Read the model definition and answer for the solid it produces. Units are mm, in the model's axes. Give positions to 0.01 mm unless a question says otherwise; leave off trailing zeros. Write each loop counter-clockwise with the first axis right and the second up, starting at its lowest first coordinate (ties: lowest second). Pieces come first, ordered by that corner, then holes. Notation, with made-up numbers: (4.25, 46.5) -> (47.25, 46.5) arc R10 cw to (47.25, 62.5) -> close; hole circle Ø6 at (-23, 53.25). An arc over 180 degrees is marked (long way). Put each result on its own line as item: value. Start each with the question number.
from build123d import *

# Parameters (mm, degrees)
SKETCH1_R           = 3.3020000000000405
BOSS_EXTRUDE1_DEPTH = 1.5875
SKETCH2_R           = 12.7
CUT_EXTRUDE1_DEPTH  = 164.69798740092241
CUT_EXTRUDE2_DEPTH  = 399.2312021708926
CUT_EXTRUDE3_DEPTH  = 399.2322845032196


with BuildPart() as part:
    # Sketch1 → Boss-Extrude1 (new body)
    with BuildSketch(Plane(origin=(-4.904e-14, 229.6997332170858, -328.0452161431734), x_dir=(1, 7e-17, -1e-16), z_dir=(0, -0.5735764363510497, 0.8191520442889892))):
        with BuildLine():
            Line((356.2998896252525, 70.55163741306428), (376.9254322382814, 80.82199071424783))
            ThreePointArc((376.9254322382814, 80.82199071424783), (382.63309358192566, 97.85145347695013), (365.6036308192234, 103.55911482059432))
            Line((365.6036308192234, 103.55911482059432), (344.97808820619434, 93.28876151941097))
            Line((344.97808820619434, 93.28876151941097), (356.2998896252525, 70.55163741306428))
        make_face()
        with Locations(Location((375.5277422986924, 94.3133905334945, 0), (0, 0, 270))):
            Circle(SKETCH1_R, mode=Mode.SUBTRACT)
    extrude(amount=BOSS_EXTRUDE1_DEPTH)

    # Sketch2 → Cut-Extrude1 (cut, through all)
    with BuildSketch(Plane(origin=(364.35174229869244, 343.62540364794484, -135.39966553044988), x_dir=(-0.9960075449626111, 0.027318171664055604, 0.08498639817338811), z_dir=(-0.0892690897094424, -0.3047987291070713, -0.9482240053685426))):
        Circle(SKETCH2_R)
    extrude(amount=CUT_EXTRUDE1_DEPTH, mode=Mode.SUBTRACT)

    # Sketch3 → Cut-Extrude2 (cut, through all)
    with BuildSketch(Plane(origin=(-4.885e-14, 228.78918062437845, -326.7448122728647), x_dir=(1, 7e-17, -1e-16), z_dir=(0, -0.5735764363510497, 0.8191520442889892))):
        with BuildLine():
            Line((359.8287026568516, 100.68352732070262), (358.4382239247449, 99.99114758047237))
            Line((358.4382239247449, 99.99114758047237), (360.8702636019665, 72.82742507790554))
            add(Edge.make_bspline(
                [(360.8702636019665, 72.82742507790554), (368.2083080665997, 89.03003410456597), (359.8287026568516, 100.68352732070262)],
                knots=[4.218717035603661, 4.218717035603661, 4.218717035603661, 5.696136664554478, 5.696136664554478, 5.696136664554478], degree=2, weights=[1, 0.7393379003717987, 1]))
        make_face()
    extrude(amount=-CUT_EXTRUDE2_DEPTH, mode=Mode.SUBTRACT)

    # Sketch4 → Cut-Extrude3 (cut, through all)
    with BuildSketch(Plane(origin=(-4.904e-14, 229.6997332170858, -328.0452161431734), x_dir=(-1, -7e-17, 1e-16), z_dir=(0, 0.5735764363510497, -0.8191520442889892))):
        with BuildLine():
            Line((-361.6174533376439, 73.19948329292563), (-360.8702636019665, 72.82742507790549))
            Line((-360.8702636019665, 72.82742507790549), (-363.361378453228, 81.54873685940132))
            add(Edge.make_bspline(
                [(-363.361378453228, 81.54873685940132), (-363.00233152155374, 77.177344146135), (-361.6174533376439, 73.19948329292563)],
                knots=[1.5208655376076283, 1.5208655376076283, 1.5208655376076283, 1.9311023959162479, 1.9311023959162479, 1.9311023959162479], degree=2, weights=[1, 0.9790368693670761, 1]))
        make_face()
    extrude(amount=-CUT_EXTRUDE3_DEPTH, mode=Mode.SUBTRACT)


solid = part.part
1) A cutting plane is placed at C-C on x = 367.75. Give the vertices of the cut face in (y, z).
2) Straight lines are drawn through the part: line 1 (X direction, y = 304.25, z = -274); line 2 (X direction, y = 309, z = -271.5); line 3 (Y direction, x = 376, z = -271.75). For each, find the intervals that lie inside material, in ascending order. Write a range as [from, to].
3) A cutting plane is placed at A-A on x = 374.75. Give the vertices of the cut face in (y, z), and give its area (3 significant figures).
4) Each of these flat-tipped pins is pushed along its axis until it touches: pin 1 Ø10 at (x, z) = (378.5, -268.5) entering from -Y; pin 2 Ø8 at (y, z) = (310, -276.5) entering from +X; pin 3 Ø5 at (y, z) = (297.5, -281.5) entering from -X; pin 4 Ø6 at (y, z) = (300, -283) entering from -X. Where does it stop, or does it pass through?
5) A cutting plane is placed at B-B on x = 370.5. Give the vertices of the cut face in (y, z), and give its area (3 significant figures).
6) For a pull along X with two mould halves and no side action, classify faces 1 (the face through (362.757, 312.92, -268.818)), 2 (the face through (372.304, 307.094, -272.898)), 3 (the face through (382.755, 309.2, -271.423)) as pulls with the +X half, pulls with the -X half, needs draft (parallel to the pull), parting line crosses it, or undercut.
Results found:
1. outline: (291.25, -283.01) -> (292.16, -284.31) -> (315.21, -268.17) -> (314.3, -266.87) -> close
2. line 1: x = [363.23, 373.11], [377.95, 383.96]
2. line 2: x = [361.66, 374.33], [376.72, 382.85]
2. line 3: y = [309.41, 310.1]
3. outline: (294.11, -281.01) -> (295.02, -282.31) -> (304.33, -275.79) -> (303.42, -274.49) -> close; (308.67, -270.81) -> (309.59, -272.11) -> (315.22, -268.16) -> (314.31, -266.86) -> close
3. area: 29.0 mm²
4. pin 1: stops at y = 304.83
4. pin 2: stops at x = 383.8
4. pin 3: stops at x = 363.18
4. pin 4: passes through
5. outline: (292.37, -282.22) -> (293.28, -283.52) -> (315.6, -267.9) -> (314.69, -266.6) -> close
5. area: 43.3 mm²
6. face 1: pulls with the -X half
6. face 2: undercut
6. face 3: parting line crosses it
